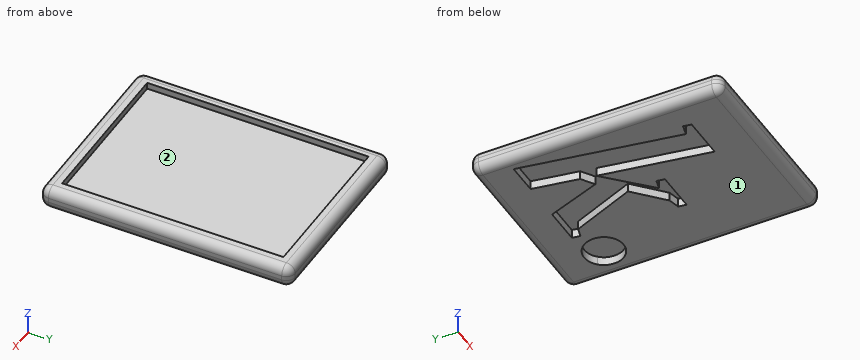
```python
from build123d import *

# Parameters (mm, degrees)
F0_W         = 108.4600649774
F0_H         = 144.723303616
F1_DEPTH     = 12.7
F2_W         = 92.2743044794
F2_H         = 127.6071891189
F3_DEPTH     = 3.81
F4_R         = 5.08
F5_T1_DEPTH  = 20.32
F5_S5_W      = 5.08
F5_S5_H      = 5.08
F5_T6_DEPTH  = 5.08
F5_S11_W     = 5.08
F5_S11_H     = 5.08
F5_T12_DEPTH = 5.08
F5_S17_W     = 5.08
F5_S17_H     = 5.08
F5_T18_DEPTH = 5.08
F5_S23_W     = 5.08
F5_S23_H     = 5.08
F5_T24_DEPTH = 5.08
F7_DEPTH     = 5.08
F8_DEPTH     = 5.08
F9_R         = 5.08


# Not quite as in the source:
# - a fillet or chamfer that OpenCascade refuses, or shapes differently, is made with other operations: its cross-section is extruded or revolved along the edge and cut away or added


with BuildPart() as f1:
    # F0 (on Top) → F1 (new body)
    with BuildSketch(Plane.XY):
        with Locations((1.0477285832, -0.3120861948)):
            Rectangle(F0_W, F0_H)
    extrude(amount=F1_DEPTH)

    # F2 (on face) → F3 (cut, symmetric)
    with BuildSketch(Plane.XY.offset(12.7)):
        with Locations((0.7300172001, -0.29200688)):
            Rectangle(F2_W, F2_H)
    extrude(amount=F3_DEPTH, both=True, mode=Mode.SUBTRACT)

    # F4
    f4_edges = [f1.edges().sort_by_distance(p)[0] for p in [
        (1.047729, 72.049566, 12.7),
        (-53.182304, -0.312086, 12.7),
        (55.277761, -0.312086, 12.7),
        (1.047729, -72.673738, 12.7),
    ]]
    fillet(f4_edges, radius=F4_R)

    # F5: fillet of radius 5.08 on 4 edges, made by hand

    # F5_s2 → F5_t1 (cut)
    with BuildSketch(Plane.XY.offset(-12.7)):
        with BuildLine():
            ThreePointArc((-48.1023039055, 72.0495656133), (-51.6944063539, 70.5616680617), (-53.1823039055, 66.9695656133))
            Line((-53.1823039055, 66.9695656133), (-53.1823039055, 72.0495656133))
            Line((-53.1823039055, 72.0495656133), (-48.1023039055, 72.0495656133))
        make_face()
        with BuildLine():
            ThreePointArc((55.2777610719, -67.5937380028), (53.7898635203, -71.1858404512), (50.1977610719, -72.6737380028))
            Line((50.1977610719, -72.6737380028), (55.2777610719, -72.6737380028))
            Line((55.2777610719, -72.6737380028), (55.2777610719, -67.5937380028))
        make_face()
        with BuildLine():
            ThreePointArc((50.1977610719, 72.0495656133), (53.7898635203, 70.5616680617), (55.2777610719, 66.9695656133))
            Line((55.2777610719, 66.9695656133), (55.2777610719, 72.0495656133))
            Line((55.2777610719, 72.0495656133), (50.1977610719, 72.0495656133))
        make_face()
        with BuildLine():
            ThreePointArc((-53.1823039055, -67.5937380028), (-51.6944063539, -71.1858404512), (-48.1023039055, -72.6737380028))
            Line((-48.1023039055, -72.6737380028), (-53.1823039055, -72.6737380028))
            Line((-53.1823039055, -72.6737380028), (-53.1823039055, -67.5937380028))
        make_face()
    extrude(amount=F5_T1_DEPTH, mode=Mode.SUBTRACT)


with BuildPart() as f5_tool4:
    # F5_s5 → F5_t6 (new body)
    with BuildSketch(Plane.YZ.offset(-48.1023039055)):
        with Locations((-70.1337380028, 10.16)):
            Rectangle(F5_S5_W, F5_S5_H)
    extrude(amount=-F5_T6_DEPTH)

    # F5_s7 → F5_t8 (revolve, cut)
    with BuildSketch(Plane(origin=(-48.1023039055, -67.5937380028, 7.62), x_dir=(0, 0.7071067812, -0.7071067812), z_dir=(0, 0.7071067812, 0.7071067812))):
        with BuildLine():
            ThreePointArc((0, -5.08), (5.08, 0), (0, 5.08))
            Line((0, 5.08), (0, -5.08))
        make_face()
    revolve(axis=Axis((-48.1023039055, -67.5937380028, 7.62), (-1, 0, 0)), mode=Mode.SUBTRACT)


with BuildPart() as f1_1:
    add(f1.part)

    # F5_t3: cut F5_tool4
    add(f5_tool4.part, mode=Mode.SUBTRACT)


with BuildPart() as f5_tool10:
    # F5_s11 → F5_t12 (new body)
    with BuildSketch(Plane.XZ.offset(-66.9695656133)):
        with Locations((52.7377610719, 10.16)):
            Rectangle(F5_S11_W, F5_S11_H)
    extrude(amount=-F5_T12_DEPTH)

    # F5_s13 → F5_t14 (revolve, cut)
    with BuildSketch(Plane(origin=(50.1977610719, 66.9695656133, 7.62), x_dir=(-0.7071067812, 0, -0.7071067812), z_dir=(0.7071067812, 0, -0.7071067812))):
        with BuildLine():
            ThreePointArc((0, -5.08), (5.08, 0), (0, 5.08))
            Line((0, 5.08), (0, -5.08))
        make_face()
    revolve(axis=Axis((50.1977610719, 66.9695656133, 7.62), (0, 1, 0)), mode=Mode.SUBTRACT)


with BuildPart() as f1_2:
    add(f1_1.part)

    # F5_t9: cut F5_tool10
    add(f5_tool10.part, mode=Mode.SUBTRACT)


with BuildPart() as f5_tool16:
    # F5_s17 → F5_t18 (new body)
    with BuildSketch(Plane.YZ.offset(50.1977610719)):
        with Locations((-70.1337380028, 10.16)):
            Rectangle(F5_S17_W, F5_S17_H)
    extrude(amount=F5_T18_DEPTH)

    # F5_s19 → F5_t20 (revolve, cut)
    with BuildSketch(Plane(origin=(50.1977610719, -67.5937380028, 7.62), x_dir=(0, 0.7071067812, -0.7071067812), z_dir=(0, -0.7071067812, -0.7071067812))):
        with BuildLine():
            ThreePointArc((0, -5.08), (5.08, 0), (0, 5.08))
            Line((0, 5.08), (0, -5.08))
        make_face()
    revolve(axis=Axis((50.1977610719, -67.5937380028, 7.62), (1, 0, 0)), mode=Mode.SUBTRACT)


with BuildPart() as f1_3:
    add(f1_2.part)

    # F5_t15: cut F5_tool16
    add(f5_tool16.part, mode=Mode.SUBTRACT)


with BuildPart() as f5_tool22:
    # F5_s23 → F5_t24 (new body)
    with BuildSketch(Plane.XZ.offset(-66.9695656133)):
        with Locations((-50.6423039055, 10.16)):
            Rectangle(F5_S23_W, F5_S23_H)
    extrude(amount=-F5_T24_DEPTH)

    # F5_s25 → F5_t26 (revolve, cut)
    with BuildSketch(Plane(origin=(-48.1023039055, 66.9695656133, 7.62), x_dir=(0.7071067812, 0, -0.7071067812), z_dir=(0.7071067812, 0, 0.7071067812))):
        with BuildLine():
            ThreePointArc((0, -5.08), (5.08, 0), (0, 5.08))
            Line((0, 5.08), (0, -5.08))
        make_face()
    revolve(axis=Axis((-48.1023039055, 66.9695656133, 7.62), (0, 1, 0)), mode=Mode.SUBTRACT)


with BuildPart() as f1_4:
    add(f1_3.part)

    # F5_t21: cut F5_tool22
    add(f5_tool22.part, mode=Mode.SUBTRACT)

    # F6 (on face) → F7 (cut)
    with BuildSketch(Plane(origin=(0, 0, 0), x_dir=(1, 0, 0), z_dir=(0, 0, -1))):
        Polygon((3.4059861085, 7.1879082529), (-20.5314729904, -16.2908951516), (-9.6110993139, 46.108120036), (-34.5313920437, 46.108120036), (-35.3613404431, 41.5870853339), (-29.0712052055, 39.9490292824), (-45.1023137626, -50.8866389588), (-26.7560859861, -50.8866389588), (-22.1040067999, -24.7432643772), (-14.7436749419, -19.9601407069), (-3.4083270657, -50.8866389588), (18.0174460877, -50.8866389588), (18.781872245, -46.3874450041), (13.3216854068, -44.7493889526), (-1.8357932562, -8.0132519048), (14.7413339847, 7.2752712423), (21.0314692224, 8.7604420623), (21.7740546324, 13.2814767644), (-1.7047487721, 13.2814767644), (-2.4473341821, 8.7604420623), align=None)
    extrude(amount=-F7_DEPTH, mode=Mode.SUBTRACT)

    # F6 (on face) → F8 (cut)
    with BuildSketch(Plane(origin=(0, 0, 0), x_dir=(1, 0, 0), z_dir=(0, 0, -1))):
        with BuildLine():
            add(Edge.make_bspline(
                [(35.2279550018, -52.874146968), (30.5103535736, -52.874146968), (27.2014803496, -49.598034865)],
                knots=[0, 0, 0, 1, 1, 1], degree=2))
            add(Edge.make_bspline(
                [(43.2653500278, -49.5543533703), (39.9892379248, -52.874146968), (35.2279550018, -52.874146968)],
                knots=[0, 0, 0, 1, 1, 1], degree=2))
            add(Edge.make_bspline(
                [(46.5414621307, -41.5387990917), (46.5414621307, -46.2345597726), (43.2653500278, -49.5543533703)],
                knots=[0, 0, 0, 1, 1, 1], degree=2))
            add(Edge.make_bspline(
                [(43.2325889067, -33.4795633185), (46.5414621307, -36.7556754214), (46.5414621307, -41.5387990917)],
                knots=[0, 0, 0, 1, 1, 1], degree=2))
            add(Edge.make_bspline(
                [(35.2279550018, -30.2034512155), (39.9237156827, -30.2034512155), (43.2325889067, -33.4795633185)],
                knots=[0, 0, 0, 1, 1, 1], degree=2))
            add(Edge.make_bspline(
                [(27.1687192286, -33.5123244395), (30.4448313315, -30.2034512155), (35.2279550018, -30.2034512155)],
                knots=[0, 0, 0, 1, 1, 1], degree=2))
            add(Edge.make_bspline(
                [(23.8926071256, -41.5387990917), (23.8926071256, -36.8211976635), (27.1687192286, -33.5123244395)],
                knots=[0, 0, 0, 1, 1, 1], degree=2))
            add(Edge.make_bspline(
                [(27.2014803496, -49.598034865), (23.8926071256, -46.321922762), (23.8926071256, -41.5387990917)],
                knots=[0, 0, 0, 1, 1, 1], degree=2))
        make_face()
    extrude(amount=-F8_DEPTH, mode=Mode.SUBTRACT)

    # F9
    f9_edges = [f1_4.edges().sort_by_distance(p)[0] for p in [
        (-51.694406, -71.18584, 0),
    ]]
    fillet(f9_edges, radius=F9_R)


solid = f1_4.part
```
Verification items for the finished model (mm, model axes). Face numbers are marked on the shaded views. Give positions to 0.01 mm unless a question says otherwise; leave off trailing zeros. Order: outer loops, then holes, each group sorted by start corner. A loop starts at its lowest first (then second) coordinate and runs counter-clockwise, first axis right, second up. Notation, with made-up numbers: M 2.25,0.5 L 50.25,0.5 A23 ccw 50.25,29.5 Z; hole C 25,-33 d7. An arc over 180 degrees is marked long. Answer in a Markdown table with one row per item. Add a question column.
Item 1: Section check A-A, the plane x = -41. Enter the section's corners in (y, z), and give its area (3 significant figures).
Item 2: Mould release check, pull along Y, two halves, no side actions. Record for the marked faces 1 and 2: released by +Y, released by -Y, zero draft, split by the parting line, or undercut.
Item 3: Gauge pin test, flat ends, axial feed: pin 1 (5.5 mm diameter, centred on x = -23.5, z = 2, fed in from +Y); pin 2 (3 mm diameter, centred on x = 8, z = 10.5, fed in from +Y); pin 3 (3 mm diameter, centred on x = -2.5, z = 10.5, fed in from -Y). Record the tip position at first contact, or that the pin passes through.
Item 4: Scan lines: probe 1 along X at (y, z) = (-10, 4.5); probe 2 along X at (y, z) = (14, 9.5); probe 3 along Z at (x, y) = (14, -56). Record each from-to range of solid material in increasing order. Write a range as from..to.
Item 5: Section check D-D, the plane x = 5. Enter the section's corners in (y, z).
Item 6: Section check C-C, the plane z = 3. State how many separate pieces and enclosed holes the cut face has, and give its area (3 significant figures).
Item 7: Section check B-B, the plane y = -3. Enter the section's corners in (x, z).
Filled sheet:
| question | item | result |
|---|---|---|
| 1 | outline | M -72.67,5.08 A5.08 ccw -67.59,0 L 27.64,0 L 27.64,5.08 L 50.89,5.08 L 50.89,0 L 66.97,0 A5.08 ccw 72.05,5.08 L 72.05,7.62 A5.08 ccw 66.97,12.7 L 63.51,12.7 L 63.51,8.89 L -64.1,8.89 L -64.1,12.7 L -67.59,12.7 A5.08 ccw -72.67,7.62 Z |
| 1 | area | 1,210 mm^2 |
| 2 | face 1 | zero draft |
| 2 | face 2 | undercut |
| 3 | pin 1 | stops at y = 72.04 |
| 3 | pin 2 | stops at y = 71.86 |
| 3 | pin 3 | stops at y = -72.48 |
| 4 | probe 1 | x = -53.15..-34.36, -15.93..-2.24, 21.24..55.24 |
| 4 | probe 2 | x = -52.82..-45.41, 46.87..54.92 |
| 4 | probe 3 | z = 0..8.89 |
| 5 | outline | M -72.67,5.08 A5.08 ccw -67.59,0 L -13.28,0 L -13.28,5.08 L 1.71,5.08 L 1.71,0 L 24.58,0 L 24.58,5.08 L 50.89,5.08 L 50.89,0 L 66.97,0 A5.08 ccw 72.05,5.08 L 72.05,7.62 A5.08 ccw 66.97,12.7 L 63.51,12.7 L 63.51,8.89 L -64.1,8.89 L -64.1,12.7 L -67.59,12.7 A5.08 ccw -72.67,7.62 Z |
| 6 | separate pieces | 1 |
| 6 | enclosed holes | 2 |
| 6 | area | 12,100 mm^2 |
| 7 | outline | M -53.18,5.08 A5.08 ccw -48.1,0 L -35.59,0 L -35.59,5.08 L -17.16,5.08 L -17.16,0 L -0.86,0 L -0.86,5.08 L 10.11,5.08 L 10.11,0 L 50.2,0 A5.08 ccw 55.28,5.08 L 55.28,7.62 A5.08 ccw 50.2,12.7 L 46.87,12.7 L 46.87,8.89 L -45.41,8.89 L -45.41,12.7 L -48.1,12.7 A5.08 ccw -53.18,7.62 Z |
